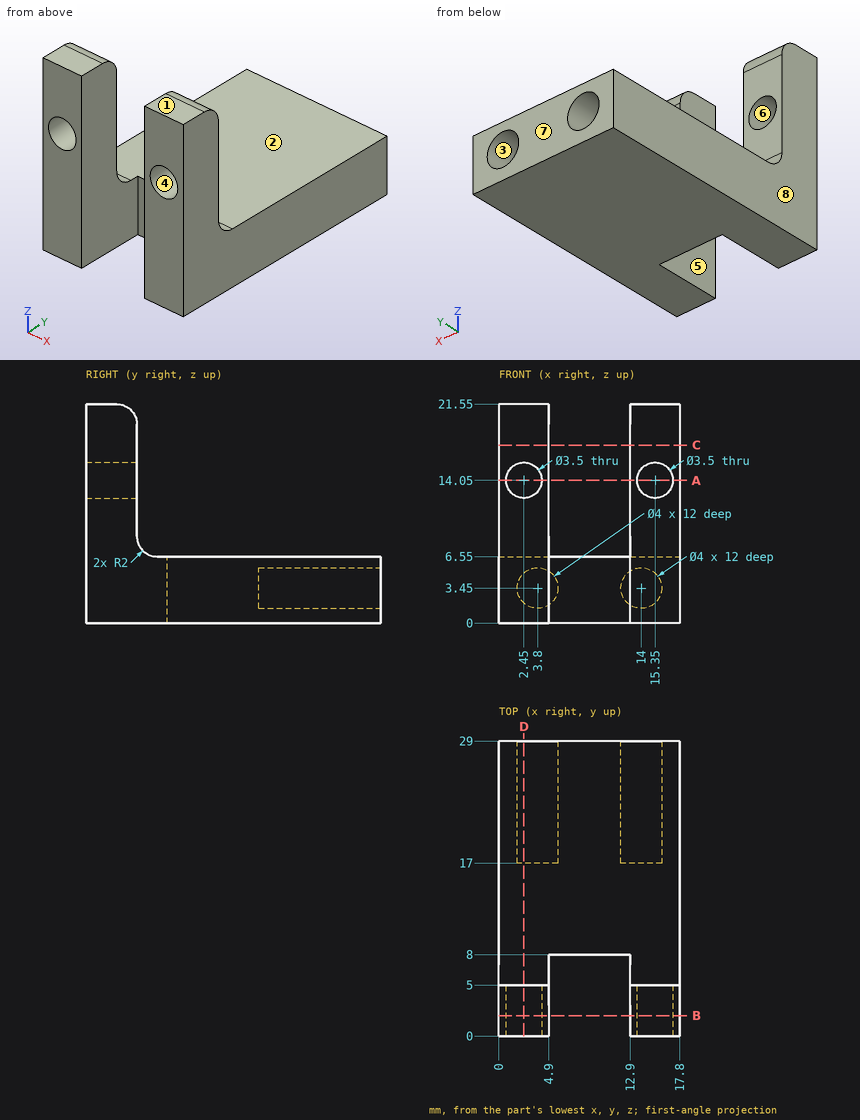
Here's the drawing with two shaded views (mm, measured from the low corner). I have some questions. A direction names the side the tool comes from. Give positions to 0.01 mm unless a question says otherwise; leave off trailing zeros. Loops run counter-clockwise (first coordinate to the right, second up) from the corner with the lowest first, then second, coordinate; pieces in that order, holes last. Notation, with made-up numbers: M 62,29 L 118,29 A27 cw 118,59 Z; hole C 18,84.25 d8. An arc over 180 degrees is marked long. Use one line per item in the form item = value. Start each with the question number.
(1) I'm going to push flat-ended pins straight in: P1, Ø1.5, axis at x = 2, y = 16, coming from the +Z side; P2, Ø6, axis at x = 4.5, z = 15, coming from the +Y side; P3, Ø2.5, axis at x = 14, z = 3.45, coming from the +Y side. Where does each tip first touch, or does it pass through?
(2) Thinking about a two-plate mould opening in X: for the marked faces 6, 7 and 8, which applies, released by +X, released by -X, zero draft, split by the parting line, or undercut?
(3) On a 3-axis mill with a long thin cutter (end or side, diameter ignored), from which of +Z, -Z, +X, -X, +Y, -Y can I reach the whole of each face in a straight line? I mean the marked faces 1, 2, 3, 4 and 5. Say none if no direction works.
(4) Please list where these lines run through material, in increasing order: line 1 (X direction, y = 1.25, z = 14.05); line 2 (X direction, y = 23, z = 3.45); line 3 (Z direction, x = 14, y = 20.25).
(5) I want a section at C-C, the plane z = 17.5. Write out the boundary of the cut face in (x, y).
(6) I want a section at B-B, the plane y = 2. Write out the boundary of the cut face in (x, z).
(7) I want a section at A-A, the plane z = 14.05. Write out the boundary of the cut face in (x, y), and give its area (3 significant figures).
(8) I want a section at D-D, the plane x = 2.45. Write out the boundary of the cut face in (y, z).
Worked out:
q1.P1 = 6.55
q1.P2 = 5
q1.P3 = 17
q2.face_6 = undercut
q2.face_7 = zero draft
q2.face_8 = released by -X
q3.face_1 = +Z, +X, -X, +Y, -Y
q3.face_2 = +Z, +X, -X, +Y
q3.face_3 = +Y
q3.face_4 = +Y, -Y
q3.face_5 = +Z, -Z, -Y
q4.line_1 = 0 to 0.7, 4.2 to 4.9, 12.9 to 13.6, 17.1 to 17.8
q4.line_2 = 0 to 1.8, 5.8 to 12, 16 to 17.8
q4.line_3 = 0 to 1.45, 5.45 to 6.55
q5.outline = M 0,0 L 4.9,0 L 4.9,5 L 0,5 Z; M 12.9,0 L 17.8,0 L 17.8,5 L 12.9,5 Z
q6.outline = M 0,0 L 4.9,0 L 4.9,21.55 L 0,21.55 Z; M 12.9,0 L 17.8,0 L 17.8,21.55 L 12.9,21.55 Z; hole C 2.45,14.05 d3.5; hole C 15.35,14.05 d3.5
q7.outline = M 0,0 L 0.7,0 L 0.7,5 L 0,5 Z; M 4.2,0 L 4.9,0 L 4.9,5 L 4.2,5 Z; M 12.9,0 L 13.6,0 L 13.6,5 L 12.9,5 Z; M 17.1,0 L 17.8,0 L 17.8,5 L 17.1,5 Z
q7.area = 14.0 mm²
q8.outline = M 0,0 L 29,0 L 29,1.97 L 17,1.97 L 17,4.93 L 29,4.93 L 29,6.55 L 7,6.55 A2 cw 5,8.55 L 5,12.3 L 0,12.3 Z; M 0,15.8 L 5,15.8 L 5,19.55 A2 ccw 3,21.55 L 0,21.55 Z
